Here's how the part is built. I have some questions about the finished solid (model axes, mm). A direction names the side the tool comes from. Round coordinates to 2 decimals unless told otherwise and drop trailing zeros. Write each loop counter-clockwise with the first axis right and the second up, starting at its lowest first coordinate (ties: lowest second). Pieces come first, ordered by that corner, then holes. Notation, with made-up numbers: (-4, -32) -> (47, -32) arc R20 ccw to (47, -3) -> close; hole circle Ø4 at (1, 36.5). An arc over 180 degrees is marked (long way). Put each result on its own line as item: value. Start each with the question number.
1. For pin 1 (4 mm diameter, centred on x = -9.525, z = -3.175, fed in from +Y); pin 2 (3 mm diameter, centred on x = 1, y = -2.5, fed in from +Z); pin 3 (12 mm diameter, centred on x = 2.5, y = 5.5, fed in from -Z), each with a flat end and sliding along its axis, tell me the tip position at first contact or that it passes through.
2. Suppose I cut it at B-B (z = 1.75). Please give me the cut outline in (x, y) (3 decimals).
3. We'd pull the mould along Y, two halves only. Please class faces 3 (the face through (2.98, 4.68, 1.57)), 4 (the face through (0, -25.908, -5)), 5 (the face through (0, -6, 0)): +Y half, -Y half, draft (parallel to the pull), parting line (faces both ways), or undercut.
4. Suppose I cut it at A-A (y = 0). Please give me the cut outline in (x, z) (3 decimals).
5. I need wall thicknesses on probe 1 along Y at (x, z) = (-5.75, 0.7) (3 decimals); probe 2 along X at (y, z) = (-24, -3.5); probe 3 along X at (y, z) = (-24, -2). Which ranges of each line are inside material? Lowest first, please. Write a range as from..to.
6. Suppose I cut it at D-D (y = -11). Please give me the cut outline in (x, z) (3 decimals).
7. Which directions (+Z, -Z, +X, -X, +Y, -Y) give clear straight access to the entire face, cutting with the end or side of a thin tool? Please do faces 1 (the face through (0, -22.733, -6)), 2 (the face through (-12.7, -13, 2)).
8. Suppose I cut it at C-C (x = -10). Please give me the cut outline in (y, z) (3 decimals), then the cut area to 3 significant figures.
```python
from build123d import *

# Parameters (mm, degrees)
SKETCH1_W                      = 25.4
SKETCH1_H                      = 35.433
SKETCH1_R                      = 5.55
BOSS_EXTRUDE1_DEPTH            = 3.175
SKETCH3_W                      = 25.4
SKETCH3_H                      = 3.175
BOSS_EXTRUDE2_DEPTH            = 12.7
FILLET1_R                      = 3.175
M2_CLEARANCE_HOLE1_D           = 2.2
F_4_CLEARANCE_HOLE1_D          = 2.9464
F_1_8_0_1250_DOWEL_HOLE1_D     = 3.175
F_1_8_0_1250_DOWEL_HOLE1_DEPTH = 4.064
F_1_8_0_1250_DOWEL_HOLE1_TIP   = 0.953866233


with BuildPart() as part:
    # Sketch1 → Boss-Extrude1 (new body)
    with BuildSketch(Plane.XY):
        with Locations((0, -8.1915)):
            Rectangle(SKETCH1_W, SKETCH1_H)
        Circle(SKETCH1_R, mode=Mode.SUBTRACT)
    extrude(amount=BOSS_EXTRUDE1_DEPTH)

    # Sketch3 → Boss-Extrude2 (add)
    with BuildSketch(Plane(origin=(0, 0, 0), x_dir=(-1, 0, 0), z_dir=(0, 0, -1))):
        with Locations((0, -24.3205)):
            Rectangle(SKETCH3_W, SKETCH3_H)
    extrude(amount=BOSS_EXTRUDE2_DEPTH)

    # Fillet1
    fillet1_edges = [part.edges().sort_by_distance(p)[0] for p in [
        (-12.7, -24.3205, -12.7),
        (12.7, -24.3205, -12.7),
        (-12.7, 9.525, 1.5875),
        (12.7, 9.525, 1.5875),
    ]]
    fillet(fillet1_edges, radius=FILLET1_R)

    # M2 Clearance Hole1 (through all)
    with Locations(Plane(origin=(0, -25.908, 3.175), x_dir=(1, 0, 0), z_dir=(0, 0, 1))):
        with Locations((5.75, 31.658), (-5.75, 31.658), (5.75, 20.158), (-5.75, 20.158)):
            Hole(M2_CLEARANCE_HOLE1_D / 2)

    # #4 Clearance Hole1 (through all)
    with Locations(Plane(origin=(0, -22.733, 0), x_dir=(1, 0, 0), z_dir=(0, 1, 0))):
        with Locations((0, 9.525)):
            Hole(F_4_CLEARANCE_HOLE1_D / 2)

    # 1/8 (0.1250) Dowel Hole1
    with Locations(Plane(origin=(0, -22.733, 0), x_dir=(1, 0, 0), z_dir=(0, 1, 0))):
        with Locations((9.525, 3.175), (-9.525, 3.175)):
            Hole(F_1_8_0_1250_DOWEL_HOLE1_D / 2, depth=F_1_8_0_1250_DOWEL_HOLE1_DEPTH)
            with Locations((0, 0, -(F_1_8_0_1250_DOWEL_HOLE1_DEPTH + F_1_8_0_1250_DOWEL_HOLE1_TIP / 2))):  # 118° drill point
                Cone(0, F_1_8_0_1250_DOWEL_HOLE1_D / 2, F_1_8_0_1250_DOWEL_HOLE1_TIP, mode=Mode.SUBTRACT)


solid = part.part
```
Verdict:
1. pin 1: stops at y = -22.73
1. pin 2: passes through
1. pin 3: stops at z = 0
2. outline: (-12.7, -25.908) -> (12.7, -25.908) -> (12.7, 6.35) arc R3.175 ccw to (9.525, 9.525) -> (-9.525, 9.525) arc R3.175 ccw to (-12.7, 6.35) -> close; hole circle Ø2.2 at (-5.75, -5.75); hole circle Ø2.2 at (-5.75, 5.75); hole circle Ø11.1 at (0, 0); hole circle Ø2.2 at (5.75, -5.75); hole circle Ø2.2 at (5.75, 5.75)
3. face 3: undercut
3. face 4: -Y half
3. face 5: draft
4. outline: (-12.7, 0) -> (-5.55, 0) -> (-5.55, 3.175) -> (-12.7, 3.175) -> close; (5.55, 0) -> (12.7, 0) -> (12.7, 3.175) -> (5.55, 3.175) -> close
5. probe 1: y = -25.908..-6.85, -4.65..4.65, 6.85..9.525
5. probe 2: x = -12.7..-11.08, -7.97..7.97, 11.08..12.7
5. probe 3: x = -12.7..-10.59, -8.46..8.46, 10.59..12.7
6. outline: (-12.7, 0) -> (12.7, 0) -> (12.7, 3.175) -> (-12.7, 3.175) -> close
7. face 1: -Z, +X, -X, +Y
7. face 2: +Z, -Z, -X, +Y, -Y
8. outline: (-25.908, -12.664) -> (-22.733, -12.664) -> (-22.733, -4.69) -> (-25.908, -4.69) -> close; (-25.908, -1.66) -> (-22.733, -1.66) -> (-22.733, 0) -> (9.489, 0) -> (9.489, 3.175) -> (-25.908, 3.175) -> close
8. area: 143 mm^2
